CAD build for the part. Positions are in the model's coordinates, mm. Give positions to 0.01 mm unless a question says otherwise; leave off trailing zeros. Write each loop counter-clockwise with the first axis right and the second up, starting at its lowest first coordinate (ties: lowest second). Pieces come first, ordered by that corner, then holes. Notation, with made-up numbers: M -24.5,-8.75 L 23.5,-8.75 A35 ccw 23.5,26.25 Z; hole C 88.5,87.25 d2. An arc over 180 degrees is marked long. One line per question, with ' | ' between items. Start each with the question number.
1. Cut at B-B, the plane z = 231.5. Write the cut outline in (x, y), then the cut area to 3 significant figures.
2. Cut at A-A, the plane y = -7. Write the cut outline in (x, z).
3. Wall check: L1, parallel to X at y = 10.5, z = 210.5; L2, parallel to Z at x = 14, y = -18.55. Give the ranges that are in metal, low to high.
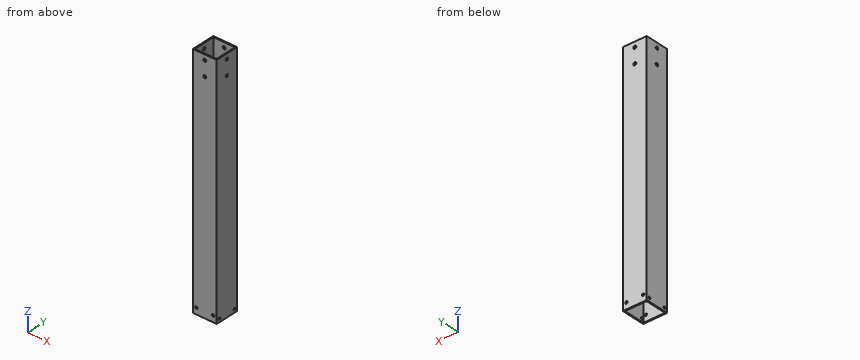
```python
from build123d import *

# Parameters (mm, degrees)
F0_W     = 40
F0_H     = 40
F0_W_2   = 36
F0_H_2   = 36
F1_DEPTH = 400
F2_R     = 2
F3_DEPTH = 40
F4_R     = 2
F5_DEPTH = 40
F6_R     = 2.5
F7_DEPTH = 40
F8_R     = 2.5
F9_DEPTH = 40


with BuildPart() as f1:
    # F0 (on Top) → F1 (new body)
    with BuildSketch(Plane.XY):
        Rectangle(F0_W, F0_H)
        Rectangle(F0_W_2, F0_H_2, mode=Mode.SUBTRACT)
    extrude(amount=F1_DEPTH)

    # F2 (on face) → F3 (cut)
    with BuildSketch(Plane.YZ.offset(20)):
        with Locations((-15, 5.5)):
            Circle(F2_R)
        with Locations((15, 5.5)):
            Circle(F2_R)
    extrude(amount=-F3_DEPTH, mode=Mode.SUBTRACT)

    # F4 (on face) → F5 (cut)
    with BuildSketch(Plane.XZ.offset(20)):
        with Locations((-14, 10.5)):
            Circle(F4_R)
        with Locations((14, 10.5)):
            Circle(F4_R)
    extrude(amount=-F5_DEPTH, mode=Mode.SUBTRACT)

    # F6 (on face) → F7 (cut)
    with BuildSketch(Plane.YZ.offset(20)):
        with Locations((0, 391.5)):
            Circle(F6_R)
        with Locations((0, 366.5)):
            Circle(F6_R)
    extrude(amount=-F7_DEPTH, mode=Mode.SUBTRACT)

    # F8 (on face) → F9 (cut)
    with BuildSketch(Plane.XZ.offset(20)):
        with Locations((0, 391.5)):
            Circle(F8_R)
        with Locations((0, 366.5)):
            Circle(F8_R)
    extrude(amount=-F9_DEPTH, mode=Mode.SUBTRACT)


solid = f1.part
```
Here are the results:
1) outline: M -20,-20 L 20,-20 L 20,20 L -20,20 Z; hole M -18,-18 L 18,-18 L 18,18 L -18,18 Z | area: 304 mm^2
2) outline: M -20,0 L -18,0 L -18,400 L -20,400 Z; M 18,0 L 20,0 L 20,400 L 18,400 Z
3) L1: -20 to -18, 18 to 20 | L2: 0 to 8.5, 12.5 to 400
